```python
from build123d import *

# Parameters (mm, degrees)
F1_DEPTH = 12.7
F2_R     = 5.08
F3_R     = 5.08


with BuildPart() as f1:
    # F0 (on Front) → F1 (new body)
    with BuildSketch(Plane.XZ):
        Polygon((-16.031148, 56.691967), (-38.766231, 56.691967), (-38.766231, -12.67918), (29.439015, -12.67918), (29.439015, 8.89), (-16.031148, 8.89), align=None)
    extrude(amount=F1_DEPTH)

    # F2
    f2_edges = [f1.edges().sort_by_distance(p)[0] for p in [
        (-38.766231, -12.7, 22.006393),
        (-27.39869, -12.7, 56.691967),
        (-16.031148, -12.7, 32.790984),
        (6.703934, -12.7, 8.89),
        (29.439015, -12.7, -1.89459),
        (-4.663608, -12.7, -12.67918),
        (29.439015, -6.35, -12.67918),
        (29.439015, -6.35, 8.89),
        (-16.031148, -6.35, 56.691967),
        (-38.766231, -6.35, 56.691967),
        (-38.766231, -6.35, -12.67918),
    ]]
    fillet(f2_edges, radius=F2_R)

    # F3
    f3_edges = [f1.edges().sort_by_distance(p)[0] for p in [
        (-4.663608, 0, -12.67918),
    ]]
    fillet(f3_edges, radius=F3_R)


solid = f1.part
```
Geometry: final body of the model. Coordinates: model frame, mm. A direction names the side the tool comes from. Give positions to 0.01 mm unless a question says otherwise; leave off trailing zeros. Write each loop counter-clockwise with the first axis right and the second up, starting at its lowest first coordinate (ties: lowest second). Pieces come first, ordered by that corner, then holes.
1. Section query C-C, the plane y = -2. Return loops of the section in (x, z).
2. Pin query (flat end, axial travel): P1, Ø1.5, axis at y = -5.5, z = 32.5, coming from the +X side; P2, Ø6, axis at y = -10.5, z = 6, coming from the +X side; P3, Ø2, axis at x = -22.5, y = -11, coming from the +Z side. Return the tip coordinate at first contact, or that it passes through.
3. Line query: probe 1 along X at (y, z) = (-5.5, 32.5); probe 2 along Y at (x, z) = (-21, 37.5); probe 3 along Z at (x, y) = (-6, -6.5). Output: solid intervals per line, ascending.
4. Section query A-A, the plane z = 47.5. Return loops of the section in (x, y), then the cut area to 3 significant figures.
5. Section query B-B, the plane x = -13.5. Return loops of the section in (y, z), then the cut area to 3 significant figures.
6. Section query D-D, the plane y = -10.75. Return loops of the section in (x, z), then the cut area to 3 significant figures.
7. Reachability of faces 1 (the cylindrical face through (-4.257, -11.172, -11.231)), 2 (the cylindrical face through (1.306, -11.172, 7.441)), 3 (the cylindrical face through (1.306, -1.449, 7.362)), 4 (the flat face through (-16.031, -6, 30)), 5 (the cylindrical face through (27.91, -1.45, -1.81)) from +Z, -Z, +X, -X, +Y, -Y: full face, straight path, thin tool, end or side. Return the list, or none.
Computed:
1. outline: (-37.73, -7.6) arc R4.04 ccw to (-33.69, -11.64) - (24.36, -11.64) arc R4.04 ccw to (28.4, -7.6) - (28.4, 3.81) arc R4.04 ccw to (24.36, 7.85) - (-17.07, 7.85) - (-17.07, 51.61) arc R4.04 ccw to (-21.11, 55.65) - (-33.69, 55.65) arc R4.04 ccw to (-37.73, 51.61) - close
2. P1: stops at x = -16.03
2. P2: stops at x = 29.4
2. P3: stops at z = 56.1
3. probe 1: x = -38.77 to -16.03
3. probe 2: y = -12.7 to 0
3. probe 3: z = -12.68 to 8.89
4. outline: (-38.77, -7.62) arc R5.08 ccw to (-33.69, -12.7) - (-21.11, -12.7) arc R5.08 ccw to (-16.03, -7.62) - (-16.03, -5.08) arc R5.08 ccw to (-21.11, 0) - (-33.69, 0) arc R5.08 ccw to (-38.77, -5.08) - close
4. area: 267 mm2
5. outline: (-12.7, -7.6) arc R5.08 ccw to (-7.62, -12.68) - (-5.08, -12.68) arc R5.08 ccw to (0, -7.6) - (0, 3.81) arc R5.08 ccw to (-5.08, 8.89) - (-7.62, 8.89) arc R5.08 ccw to (-12.7, 3.81) - close
5. area: 252 mm2
6. outline: (-37.69, -7.6) arc R4 ccw to (-33.69, -11.6) - (24.36, -11.6) arc R4 ccw to (28.36, -7.6) - (28.36, 3.81) arc R4 ccw to (24.36, 7.81) - (-17.11, 7.81) - (-17.11, 51.61) arc R4 ccw to (-21.11, 55.61) - (-33.69, 55.61) arc R4 ccw to (-37.69, 51.61) - close
6. area: 2,250 mm2
7. face 1: -Z, +X, -X, -Y
7. face 2: +Z, +X, -Y
7. face 3: +Z, +X, +Y
7. face 4: +Z, +X, +Y, -Y
7. face 5: +Z, -Z, +X, +Y
